Can you work these out from the model? Positions are in its coordinate system, mm. Give positions to 0.01 mm unless a question says otherwise; leave off trailing zeros. Answer as CSV lines item,"result".
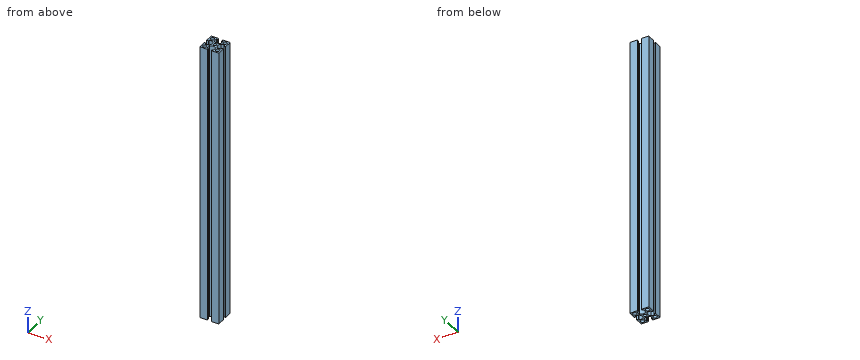
```python
from build123d import *

# Parameters (mm, degrees)
F0_R     = 3
F0_R_2   = 2.5
F1_DEPTH = 445


with BuildPart() as f1:
    # F0 (on Top) → F1 (new body)
    with BuildSketch(Plane.XY):
        with BuildLine():
            Line((-15, 15), (-15, 3.15))
            Line((-15, 3.15), (-12.5, 3.15))
            Line((-12.5, 3.15), (-12.5, 5.15))
            Line((-12.5, 5.15), (-6.547707, 5.15))
            ThreePointArc((-6.547707, 5.15), (-4.5, 0), (-6.547707, -5.15))
            Line((-6.547707, -5.15), (-12.5, -5.15))
            Line((-12.5, -5.15), (-12.5, -3.15))
            Line((-12.5, -3.15), (-15, -3.15))
            Line((-15, -3.15), (-15, -15))
            Line((-15, -15), (-3.15, -15))
            Line((-3.15, -15), (-3.15, -12.5))
            Line((-3.15, -12.5), (-5.15, -12.5))
            Line((-5.15, -12.5), (-5.15, -6.547707))
            ThreePointArc((-5.15, -6.547707), (0, -4.5), (5.15, -6.547707))
            Line((5.15, -6.547707), (5.15, -12.5))
            Line((5.15, -12.5), (3.15, -12.5))
            Line((3.15, -12.5), (3.15, -15))
            Line((3.15, -15), (15, -15))
            Line((15, -15), (15, -3.15))
            Line((15, -3.15), (12.5, -3.15))
            Line((12.5, -3.15), (12.5, -5.15))
            Line((12.5, -5.15), (6.547707, -5.15))
            ThreePointArc((6.547707, -5.15), (4.5, 0), (6.547707, 5.15))
            Line((6.547707, 5.15), (12.5, 5.15))
            Line((12.5, 5.15), (12.5, 3.15))
            Line((12.5, 3.15), (15, 3.15))
            Line((15, 3.15), (15, 15))
            Line((15, 15), (3.15, 15))
            Line((3.15, 15), (3.15, 12.5))
            Line((3.15, 12.5), (5.15, 12.5))
            Line((5.15, 12.5), (5.15, 6.547707))
            ThreePointArc((5.15, 6.547707), (0, 4.5), (-5.15, 6.547707))
            Line((-5.15, 6.547707), (-5.15, 12.5))
            Line((-5.15, 12.5), (-3.15, 12.5))
            Line((-3.15, 12.5), (-3.15, 15))
            Line((-3.15, 15), (-15, 15))
        make_face()
        with Locations((-10, -10)):
            Circle(F0_R, mode=Mode.SUBTRACT)
        with Locations((10, -10)):
            Circle(F0_R, mode=Mode.SUBTRACT)
        with Locations((-10, 10)):
            Circle(F0_R, mode=Mode.SUBTRACT)
        Circle(F0_R_2, mode=Mode.SUBTRACT)
        with Locations((10, 10)):
            Circle(F0_R, mode=Mode.SUBTRACT)
    extrude(amount=F1_DEPTH)


solid = f1.part
```
Item 1: For pin 1 (1.5 mm diameter, centred on x = -10, y = -4, fed in from +Z); pin 2 (1.5 mm diameter, centred on x = 1.5, z = 179, fed in from +Y); pin 3 (1.5 mm diameter, centred on y = 0, z = 166.5, fed in from -X), each with a flat end and sliding along its axis, tell me the tip position at first contact or that it passes through.
Numbers:
pin 1,"passes through"
pin 2,"stops at y = 4.85"
pin 3,"stops at x = -4.54"
Item 2: Please list where these lines run through material, in increasing order: line 1 along Y through (x, z) = (10.5, 189); line 2 along X through (y, z) = (9.75, 351.5); line 3 along Y through (x, z) = (6.75, 153).
Numbers:
line 1,"y = -15 to -12.96, -7.04 to -5.15, 5.15 to 7.04, 12.96 to 15"
line 2,"x = -15 to -12.99, -7.01 to -5.15, 5.15 to 7.01, 12.99 to 15"
line 3,"y = -15 to -5.15, 5.15 to 15"
Item 3: Imagine slicing it at A-A, the plane z = 280. Give the number of separate pieces and of enclosed holes in the cut face, then the cut area to 3 significant figures.
Numbers:
separate pieces,"1"
enclosed holes,"5"
area,"401 mm²"
